```python
from build123d import *

# Parameters (mm, degrees)
SKETCH1_R           = 4.1656
BOSS_EXTRUDE2_DEPTH = 6.35


with BuildPart() as part:
    # Sketch1 → Boss-Extrude2 (new body)
    with BuildSketch(Plane(origin=(0, 0, 0), x_dir=(1, 0, 0), z_dir=(0, 1, 0))):
        with BuildLine():
            Line((-77.22358209, -17.628358209), (-77.22358209, 20.471641791))
            Line((-77.22358209, 20.471641791), (-45.47358209, 20.471641791))
            ThreePointArc((-45.47358209, 20.471641791), (-40.983454029, 22.331513731), (-39.12358209, 26.821641791))
            Line((-39.12358209, 26.821641791), (-39.12358209, 96.671641791))
            Line((-39.12358209, 96.671641791), (-1.02358209, 96.671641791))
            Line((-1.02358209, 96.671641791), (-1.02358209, 26.821641791))
            ThreePointArc((-1.02358209, 26.821641791), (0.83628985, 22.331513731), (5.32641791, 20.471641791))
            Line((5.32641791, 20.471641791), (37.07641791, 20.471641791))
            Line((37.07641791, 20.471641791), (37.07641791, -17.628358209))
            Line((37.07641791, -17.628358209), (-77.22358209, -17.628358209))
        make_face()
        with Locations(Location((-20.07358209, 77.621641791, 0), (0, 0, 270))):
            Circle(SKETCH1_R, mode=Mode.SUBTRACT)
        with Locations(Location((-20.07358209, 39.521641791, 0), (0, 0, 270))):
            Circle(SKETCH1_R, mode=Mode.SUBTRACT)
        with Locations(Location((-20.07358209, 1.421641791, 0), (0, 0, 270))):
            Circle(SKETCH1_R, mode=Mode.SUBTRACT)
        with Locations(Location((18.02641791, 1.421641791, 0), (0, 0, 270))):
            Circle(SKETCH1_R, mode=Mode.SUBTRACT)
        with Locations(Location((-58.17358209, 1.421641791, 0), (0, 0, 270))):
            Circle(SKETCH1_R, mode=Mode.SUBTRACT)
    extrude(amount=BOSS_EXTRUDE2_DEPTH)


solid = part.part
```
Design review of the part built by this model. Coordinates are the model's own, in mm. A direction names the side the tool comes from. Give positions to 0.01 mm unless a question says otherwise; leave off trailing zeros. Loops run counter-clockwise (first coordinate to the right, second up) from the corner with the lowest first, then second, coordinate; pieces in that order, holes last. Notation, with made-up numbers: M 53.5,-5.5 L 84.5,-5.5 A12 cw 84.5,11.5 Z; hole C -21,62 d2. An arc over 180 degrees is marked long. Return JSON: item names as keys, results as strings. Group by question number.
Item 1: Insertion check: pin 1 Ø3 at (y, z) = (4, -74) entering from +X; pin 2 Ø3 at (x, y) = (22, 2) entering from -Z. Each pin has a flat end and moves straight along its axis. Give the tip position at first contact, or say it passes through.
Item 2: We need section D-D (z = -63). Give the boundary of the cut face in (x, y).
Item 3: We need section A-A (z = -76). Give the boundary of the cut face in (x, y).
Item 4: We need section C-C (y = 4). Give the boundary of the cut face in (x, z), and give its area (3 significant figures).
Item 5: For probe 1 along Z at (x, y) = (-22, 3.25); probe 2 along Z at (x, y) = (-45, 2); probe 3 along Z at (x, y) = (-59, 1.75), list the stretches that pass through material, from the lowest coordinate up.
Item 6: Tool access review of faces 1 (the cylindrical face through (-15.943, 3.131, -1.964)), 2 (the flat face through (-62, 3, -20.472)), 3 (the flat face through (-1.024, 3, -62)): name each direction out of +Z, -Z, +X, -X, +Y, -Y from which nothing blocks a thin tool from reaching the whole face with its end or side.
Item 7: Mouldability with a two-part tool opening along Z and no side actions: class faces 4 (the cylindrical face through (-19.89, 3.131, -81.783)), 5 (the flat face through (21, 3, -20.472)), 6 (the cylindrical face through (-54.043, 3.131, -1.964)), 7 (the flat face through (-39.124, 3, -61)) as released by +Z, released by -Z, zero draft, split by the parting line, or undercut.
Item 8: We need section B-B (x = -56). Give the boundary of the cut face in (y, z), and give its area (3 significant figures).
Output:
{
 "1": {"pin 1": "stops at x = -1.02", "pin 2": "stops at z = -20.47"},
 "2": {"outline": "M -39.12,0 L -1.02,0 L -1.02,6.35 L -39.12,6.35 Z"},
 "3": {"outline": "M -39.12,0 L -23.91,0 L -23.91,6.35 L -39.12,6.35 Z; M -16.24,0 L -1.02,0 L -1.02,6.35 L -16.24,6.35 Z"},
 "4": {"outline": "M -77.22,-20.47 L -45.47,-20.47 A6.35 cw -39.12,-26.82 L -39.12,-96.67 L -1.02,-96.67 L -1.02,-26.82 A6.35 cw 5.33,-20.47 L 37.08,-20.47 L 37.08,17.63 L -77.22,17.63 Z; hole C -58.17,-1.42 d8.33; hole C -20.07,-77.62 d8.33; hole C -20.07,-39.52 d8.33; hole C -20.07,-1.42 d8.33; hole C 18.03,-1.42 d8.33", "area": "7,000 mm^2"},
 "5": {"probe 1": "z = -96.67 to -81.32, -73.93 to -43.22, -35.83 to -5.12, 2.27 to 17.63", "probe 2": "z = -20.49 to 17.63", "probe 3": "z = -20.47 to -5.5, 2.66 to 17.63"},
 "6": {"face 1": "+Y, -Y", "face 2": "-Z, -X, +Y, -Y", "face 3": "-Z, +X, +Y, -Y"},
 "7": {"face 4": "undercut", "face 5": "released by -Z", "face 6": "undercut", "face 7": "zero draft"},
 "8": {"outline": "M 0,-20.47 L 6.35,-20.47 L 6.35,-4.98 L 0,-4.98 Z; M 0,2.13 L 6.35,2.13 L 6.35,17.63 L 0,17.63 Z", "area": "197 mm^2"}
}
